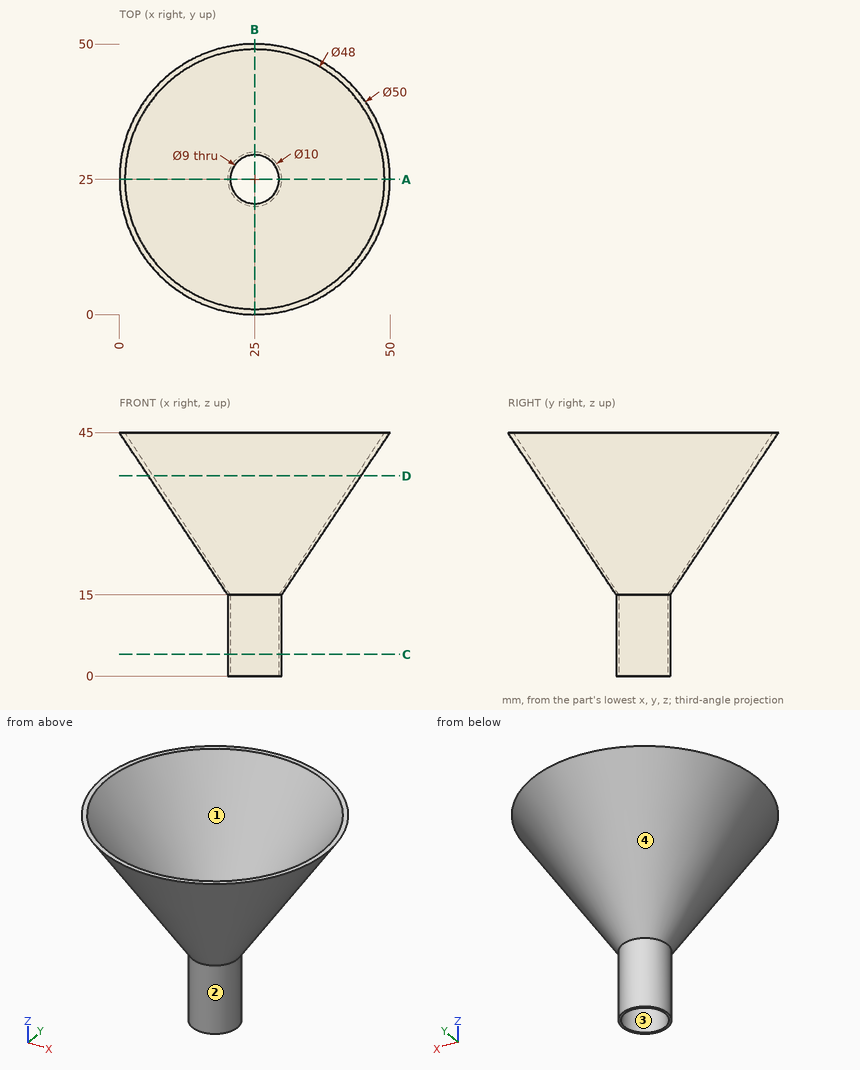
Part print with two shaded views. Sizes in mm from the minimum x, y, z corner. A direction names the side the tool comes from. Give positions to 0.01 mm unless a question says otherwise; leave off trailing zeros. Order: outer loops, then holes, each group sorted by start corner. A loop starts at its lowest first (then second) coordinate and runs counter-clockwise, first axis right, second up. Notation, with made-up numbers: (6.5, 1.25) - (26.5, 1.25) arc R22 ccw to (26.5, 33.25) - close; hole circle Ø2 at (88.25, -13). An arc over 180 degrees is marked (long way). Write each question's results on one line, items separated by ' | '.
1. Saw through at C-C on z = 4. List the corners of the cut face in (x, y).
Calculated:
outline: circle Ø10 at (25, 25); hole circle Ø9 at (25, 25)
2. Saw through at D-D on z = 37. List the corners of the cut face in (x, y).
Calculated:
outline: circle Ø39.33 at (25, 25); hole circle Ø37.6 at (25, 25)
3. Pull direction Y, two halves, no side cores. Call the marked faces 3 and 4: released by +Y, released by -Y, zero draft, split by the parting line, or undercut.
Calculated:
face 3: undercut | face 4: split by the parting line
4. Saw through at A-A on y = 25. List the corners of the cut face in (x, z).
Calculated:
outline: (0, 45) - (20, 15) - (20, 0) - (20.5, 0) - (20.5, 15) - (1, 45) - close; (29.5, 0) - (30, 0) - (30, 15) - (50, 45) - (49, 45) - (29.5, 15) - close
5. Probe L1, parallel to Y at x = 25, z = 7; L2, parallel to Y at x = 30, z = 38; L3, parallel to X at y = 19, z = 30. List the from-to ranges inside material, lowest first. Write a range as from..to.
Calculated:
L1: y = 20..20.5, 29.5..30 | L2: y = 5.29..6.2, 43.8..44.71 | L3: x = 11.25..12.07, 37.93..38.75
6. 3-axis set-ups, long thin cutter, end or side, ignore diameter. For the marked faces 1 and 2: which of +Z, -Z, +X, -X, +Y, -Y reach the whole face in a straight line?
Calculated:
face 1: +Z | face 2: -Z
7. Pin check, flat tips, straight feed: pin 1 (2 mm diameter, centred on x = 39.5, y = 37.5, fed in from -Z); pin 2 (1.5 mm diameter, centred on x = 21.5, y = 8.5, fed in from +Z); pin 3 (14.5 mm diameter, centred on x = 25, y = 25, fed in from +Z). Stop position of each tip, or through.
Calculated:
pin 1: stops at z = 34.72 | pin 2: stops at z = 35.18 | pin 3: stops at z = 19.23
